from build123d import *

# Parameters (mm, degrees)
F0_R     = 2.55
F1_DEPTH = 9
F2_DEPTH = 0.8
F4_DEPTH = 9
F7_DEPTH = 9


with BuildPart() as f1:
    # F0 (on Right) → F1 (new body)
    with BuildSketch(Plane.YZ):
        with BuildLine():
            ThreePointArc((-26.7124370169, 10.1882511594), (-26.3563013281, 6.3563288866), (-22.5219113781, 6.0278252414))
            ThreePointArc((-22.5219113781, 6.0278252414), (-21.875519954, 6.6422568398), (-21.4383157397, 7.4195602151))
            ThreePointArc((-21.4383157397, 7.4195602151), (-21.2919649304, 7.9435133623), (-21.2426406871, 8.4852813742))
            ThreePointArc((-21.2426406871, 8.4852813742), (-22.8478126252, 11.1413037156), (-25.9456104723, 10.9550777041))
            ThreePointArc((-25.9456104723, 10.9550777041), (-26.2048620049, 10.447502692), (-26.7124370169, 10.1882511594))
        make_face()
        with Locations((-24.2426406871, 8.4852813742)):
            Circle(F0_R, mode=Mode.SUBTRACT)
        with BuildLine():
            Line((-24.6525061657, 4.5359667102), (-22.5219113781, 6.0278252414))
            ThreePointArc((-22.5219113781, 6.0278252414), (-26.3563013281, 6.3563288866), (-26.7124370169, 10.1882511594))
            ThreePointArc((-26.7124370169, 10.1882511594), (-27.5629018113, 11.7016238155), (-25.9339357775, 11.1015764646))
            ThreePointArc((-25.9339357775, 11.1015764646), (-25.9368590705, 11.0280948592), (-25.9456104723, 10.9550777041))
            ThreePointArc((-25.9456104723, 10.9550777041), (-22.8478126252, 11.1413037156), (-21.2426406871, 8.4852813742))
            ThreePointArc((-21.2426406871, 8.4852813742), (-21.2919649304, 7.9435133623), (-21.4383157397, 7.4195602151))
            Line((-21.4383157397, 7.4195602151), (-18.7531459804, 14.4852813742))
            Line((-18.7531459804, 14.4852813742), (-29.6213270116, 14.4852813742))
            Line((-29.6213270116, 14.4852813742), (-36, 10.018886464))
            Line((-36, 10.018886464), (-36, -5.7573593129))
            Line((-36, -5.7573593129), (-20, -5.7573593129))
            Line((-20, -5.7573593129), (-9.7573593129, -5.7573593129))
            Line((-9.7573593129, -5.7573593129), (-9.7573593129, -5.3786863245))
            Line((-9.7573593129, -5.3786863245), (-9.7573593129, 5.4894947067))
            Line((-9.7573593129, 5.4894947067), (-16.823080472, 2.8043249475))
            ThreePointArc((-16.823080472, 2.8043249475), (-14.0540043113, 2.4695306718), (-12.7573593129, 0))
            ThreePointArc((-12.7573593129, 0), (-12.8929755232, -0.8917990274), (-13.2875629831, -1.7029697852))
            ThreePointArc((-13.2875629831, -1.7029697852), (-12.5410168717, -1.9123290566), (-12.2160642225, -2.6162950904))
            ThreePointArc((-12.2160642225, -2.6162950904), (-13.2145458279, -3.5383717974), (-14.0543895277, -2.4697963298))
            ThreePointArc((-14.0543895277, -2.4697963298), (-17.8863118005, -2.113660641), (-18.2148154457, 1.7207293091))
            Line((-18.2148154457, 1.7207293091), (-19.7066739769, -0.4098654786))
            ThreePointArc((-19.7066739769, -0.4098654786), (-21.9026628816, -1.6777202638), (-24.2854504534, -0.8104565131))
            Line((-24.2854504534, -0.8104565131), (-25.0530972002, -0.0428097662))
            ThreePointArc((-25.0530972002, -0.0428097662), (-25.9203609509, 2.3399778056), (-24.6525061657, 4.5359667102))
        make_face()
        with BuildLine():
            ThreePointArc((-16.823080472, 2.8043249475), (-17.6003838473, 2.3671207332), (-18.2148154457, 1.7207293091))
            ThreePointArc((-18.2148154457, 1.7207293091), (-17.8863118005, -2.113660641), (-14.0543895277, -2.4697963298))
            ThreePointArc((-14.0543895277, -2.4697963298), (-13.7951379951, -1.9622213178), (-13.2875629831, -1.7029697852))
            ThreePointArc((-13.2875629831, -1.7029697852), (-12.8929755232, -0.8917990274), (-12.7573593129, 0))
            ThreePointArc((-12.7573593129, 0), (-14.0540043113, 2.4695306718), (-16.823080472, 2.8043249475))
        make_face()
        with Locations((-15.7573593129, 0)):
            Circle(F0_R, mode=Mode.SUBTRACT)
    extrude(amount=F1_DEPTH)

    # F0 (on Right) → F2 (join)
    with BuildSketch(Plane.YZ):
        with Locations((-15.7573593129, 0)):
            Circle(F0_R)
        with Locations((-24.2426406871, 8.4852813742)):
            Circle(F0_R)
        with BuildLine():
            ThreePointArc((-25.9456104723, 10.9550777041), (-26.3639610307, 10.6066017178), (-26.7124370169, 10.1882511594))
            ThreePointArc((-26.7124370169, 10.1882511594), (-26.2048620049, 10.447502692), (-25.9456104723, 10.9550777041))
        make_face()
        with BuildLine():
            ThreePointArc((-25.9339357775, 11.1015764646), (-27.5629018113, 11.7016238155), (-26.7124370169, 10.1882511594))
            ThreePointArc((-26.7124370169, 10.1882511594), (-26.3639610307, 10.6066017178), (-25.9456104723, 10.9550777041))
            ThreePointArc((-25.9456104723, 10.9550777041), (-25.9368590705, 11.0280948592), (-25.9339357775, 11.1015764646))
        make_face()
        with BuildLine():
            ThreePointArc((-13.2875629831, -1.7029697852), (-13.7951379951, -1.9622213178), (-14.0543895277, -2.4697963298))
            ThreePointArc((-14.0543895277, -2.4697963298), (-13.6360389693, -2.1213203436), (-13.2875629831, -1.7029697852))
        make_face()
        with BuildLine():
            ThreePointArc((-13.2875629831, -1.7029697852), (-13.6360389693, -2.1213203436), (-14.0543895277, -2.4697963298))
            ThreePointArc((-14.0543895277, -2.4697963298), (-13.2145458279, -3.5383717974), (-12.2160642225, -2.6162950904))
            ThreePointArc((-12.2160642225, -2.6162950904), (-12.5410168717, -1.9123290566), (-13.2875629831, -1.7029697852))
        make_face()
    extrude(amount=F2_DEPTH)

    # F3 (on face) → F4 (join, through all)
    with BuildSketch(Plane.YZ):
        Polygon((-20, -5.7573593129), (-36, -5.7573593129), (-36, -15.7573593129), (-19.7573593129, -15.7573593129), (-9.7573593129, -5.7573593129), align=None)
    extrude(amount=F4_DEPTH)

    # F6 (on face) → F7 (join, through all)
    with BuildSketch(Plane.YZ.offset(9)):
        Polygon((-9.7573593129, -15.7573593129), (-14.7573593129, -10.7573593129), (-19.7573593129, -15.7573593129), align=None)
    extrude(amount=-F7_DEPTH)


solid = f1.part
Build history of the part. All positions in model axes, mm. A direction names the side the tool comes from. Round coordinates to 2 decimals unless told otherwise and drop trailing zeros. Loops run counter-clockwise (first coordinate to the right, second up) from the corner with the lowest first, then second, coordinate; pieces in that order, holes last. Notation, with made-up numbers: (-3.5, 0) -> (27.5, 0) arc R10 ccw to (27.5, 12) -> close; hole circle Ø10 at (15, 0.25). An arc over 180 degrees is marked (long way). Use CSV: the item, a comma, the result in double quotes. Start each with the question number.
Q1. Drill centre lines: L1, parallel to Z at x = 3.25, y = -13.5; L2, parallel to Z at x = 5.5, y = -22; L3, parallel to Y at x = 5.25, z = -1. Where is each one in solid material? Low to high.
Q2. Saw through at C-C on z = 11.5. Give the cut face in (x, y), and give its area (3 significant figures).
Q3. Flat gauge pins, fed straight in: pin 1 Ø0.9 at (y, z) = (-27, 11) entering from +X; pin 2 Ø2 at (x, y) = (1.5, -13.5) entering from +Z; pin 3 Ø1.5 at (x, z) = (6, 6.5) entering from +Y. Where does each tip first touch, or does it go through?
Q4. Saw through at A-A on x = 2.75. Count the separate pieces of the cut face and the enclosed holes in it, and give its area (3 significant figures).
Q5. Saw through at B-B on z = -9. Give the cut face in (x, y), and give its area (3 significant figures).
Q6. Mould opens along Z. For faces 1 (the face through (5, -23, -15.757)), 2 (the face through (4.437, -17.59, 2.375)), 3 (the face through (4.437, -21.866, -1.674)) say: +Z half, -Z half, draft (parallel to the pull), parting line (faces both ways), or undercut.
Q7. Which spindle directions (+Z, -Z, +X, -X, +Y, -Y) get a long thin tool onto all of the face, cutting with end or side? Do faces 4 (the face through (4.437, -25.923, 2.303)), 5 (the face through (0.8, -24, 9)), 6 (the face through (4.437, -13.241, 4.166)), 7 (the face through (4.437, -21.883, 6.632)), 8 (the face through (9, -26, -4)). Say none if no direction does.
Solutions:
1,L1,"z = -15.76 to -12.01, -9.5 to -3.47, -1.76 to -1.19, 1.19 to 4.07"
1,L2,"z = -15.76 to -1.68, 6.49 to 7.27, 9.7 to 14.49"
1,L3,"y = -36 to -24.08, -20.25 to -18.1, -13.41 to -9.76"
2,outline,"(0, -33.88) -> (9, -33.88) -> (9, -27.69) -> (0.8, -27.69) -> (0.8, -26.02) -> (9, -26.02) -> (9, -19.89) -> (0, -19.89) -> close"
2,area,"112 mm^2"
3,pin 1,"stops at x = 0.8"
3,pin 2,"stops at z = 4.45"
3,pin 3,"stops at y = -21.51"
4,separate pieces,"1"
4,enclosed holes,"4"
4,area,"553 mm^2"
5,outline,"(0, -36) -> (9, -36) -> (9, -13) -> (0, -13) -> close"
5,area,"207 mm^2"
6,face 1,"-Z half"
6,face 2,"+Z half"
6,face 3,"undercut"
7,face 4,"+X, -X"
7,face 5,"+X"
7,face 6,"+Z, +X, -X"
7,face 7,"+X, -X, +Y"
7,face 8,"+Z, -Z, +X, +Y, -Y"
